Geometry: final body of the model. Coordinates: model frame, mm. Face numbers are marked on the shaded views. A direction names the side the tool comes from. Give positions to 0.01 mm unless a question says otherwise; leave off trailing zeros. Order: outer loops, then holes, each group sorted by start corner. A loop starts at its lowest first (then second) coordinate and runs counter-clockwise, first axis right, second up. Notation, with made-up numbers: (65, 49.5) - (100, 49.5) arc R22 ccw to (100, 59.5) - close; hole circle Ø7 at (-26, 10). An arc over 180 degrees is marked (long way). Put each result on its own line as item: value. Start each with the question number.
1. Section C-C on y = 0. Return the cut outline in (x, z).
2. Mould query, pull axis Y, two halves, no side actions, for the marked faces 4, 5 and 6. Classes: pulls with the +Y half, pulls with the -Y half, needs draft (parallel to the pull), parting line crosses it, or undercut.
3. First-contact query: P1, Ø0.8, axis at y = 2, z = 0.5, coming from the -X side. Flat tip, straight axial feed; report the tip coordinate or a pass-through.
4. Section B-B on x = -4. Return the cut outline in (y, z).
5. Ray query, line 1 along X through (y, z) = (-0.85, 0.1); line 2 along X through (y, z) = (-0.8, 1.35); line 3 along Y through (x, z) = (4, 1.5). Return the intervals inside material, ascending. Write a range as from..to.
6. Section A-A on y = 1.7. Return the cut outline in (x, z), plus the area to 3 significant figures.
7. Section D-D on z = 1.3. Return the cut outline in (x, y).
8. Set-up query: the marked faces 1, 2 and 3. Return all of +Z, -Z, +X, -X, +Y, -Y with unobstructed straight access to the full face (end or side cutting, diameter ignored); none if empty.
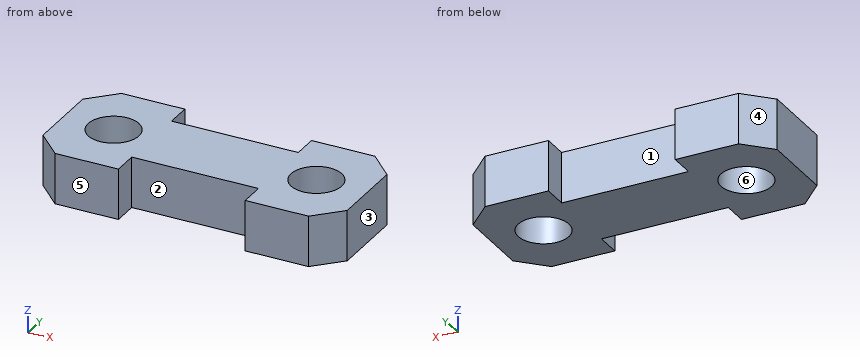
from build123d import *

# Parameters (mm, degrees)
SKETCH_1_R      = 1
EXTRUDE_1_DEPTH = 2


with BuildPart() as part:
    # 草图1 → 凸台-拉伸1 (new body)
    with BuildSketch(Plane.XY):
        Polygon((-2.5, 2.5), (-2.5, 1.5), (2.5, 1.5), (2.5, 2.5), (5, 2.5), (6, 1.5), (6, -1.5), (5, -2.5), (2.5, -2.5), (2.5, -1.5), (-2.5, -1.5), (-2.5, -2.5), (-5, -2.5), (-6, -1.5), (-6, 1.5), (-5, 2.5), align=None)
        with Locations((-4, 0)):
            Circle(SKETCH_1_R, mode=Mode.SUBTRACT)
        with Locations((4, 0)):
            Circle(SKETCH_1_R, mode=Mode.SUBTRACT)
    extrude(amount=EXTRUDE_1_DEPTH)


solid = part.part
Resolved:
1. outline: (-6, 0) - (-5, 0) - (-5, 2) - (-6, 2) - close; (-3, 0) - (3, 0) - (3, 2) - (-3, 2) - close; (5, 0) - (6, 0) - (6, 2) - (5, 2) - close
2. face 4: pulls with the +Y half
2. face 5: pulls with the -Y half
2. face 6: undercut
3. P1: x = -5.9
4. outline: (-2.5, 0) - (-1, 0) - (-1, 2) - (-2.5, 2) - close; (1, 0) - (2.5, 0) - (2.5, 2) - (1, 2) - close
5. line 1: -6..-4.53, -3.47..3.47, 4.53..6
5. line 2: -6..-4.6, -3.4..3.4, 4.6..6
5. line 3: -2.5..-1, 1..2.5
6. outline: (-5.8, 0) - (-2.5, 0) - (-2.5, 2) - (-5.8, 2) - close; (2.5, 0) - (5.8, 0) - (5.8, 2) - (2.5, 2) - close
6. area: 13.2 mm^2
7. outline: (-6, -1.5) - (-5, -2.5) - (-2.5, -2.5) - (-2.5, -1.5) - (2.5, -1.5) - (2.5, -2.5) - (5, -2.5) - (6, -1.5) - (6, 1.5) - (5, 2.5) - (2.5, 2.5) - (2.5, 1.5) - (-2.5, 1.5) - (-2.5, 2.5) - (-5, 2.5) - (-6, 1.5) - close; hole circle Ø2 at (-4, 0); hole circle Ø2 at (4, 0)
8. face 1: +Z, -Z, +Y
8. face 2: +Z, -Z, -Y
8. face 3: +Z, -Z, +X, +Y, -Y
